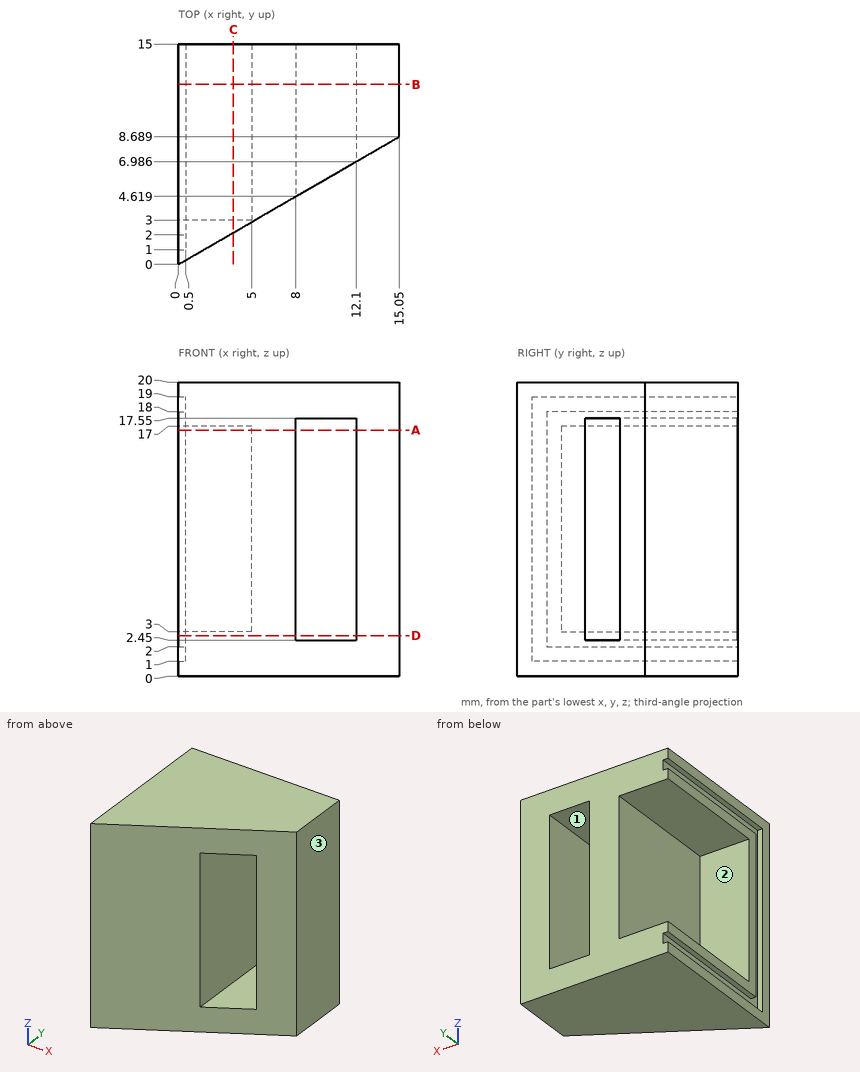
Answer from the drawing. Dimensions are ordinates in mm from the lowest x, y and z of the part. A direction names the side the tool comes from. Coordinates: 2 decimals unless noted, no trailing zeros. Loops run counter-clockwise (first coordinate to the right, second up) from the corner with the lowest first, then second, coordinate; pieces in that order, holes last. Notation, with made-up numbers: (-3, -32.5) - (35, -32.5) arc R8 ccw to (35, -22.5) - close; hole circle Ø8 at (-29, -4.75). An arc over 180 degrees is marked (long way). Answer in a Markdown table with one row per item.
1. Which of the six approach directions +Z, -Z, +X, -X, +Y, -Y give full straight-line access (tool end or side, diameter ignored) to the marked faces 1, 2 and 3?
Conclusion:
| item | result |
|---|---|
| face 1 | +Y, -Y |
| face 2 | -X, +Y |
| face 3 | +Z, -Z, +X, +Y, -Y |
2. Find section C-C, the plane x = 3.75. Write down the section's boundary in (y, z) (3 decimals), then the cut area to 3 significant figures.
Conclusion:
| item | result |
|---|---|
| outline | (2.165, 0) - (15, 0) - (15, 3) - (3, 3) - (3, 17) - (15, 17) - (15, 20) - (2.165, 20) - close |
| area | 88.7 mm² |
3. Given pin 1 (1 mm diameter, centred on y = 3, z = 3, fed in from -X); pin 2 (6.5 mm diameter, centred on y = 9.5, z = 13.5, fed in from -X); pin 3 (2 mm diameter, centred on x = 3, z = 12.5, fed in from +Y); pin 4 (1 mm diameter, centred on y = 2.5, z = 12.5, fed in from +X) (1 decimal), each flat-ended and moving along its own axis, determine where each tip first touches the part or whether it passes through.
Conclusion:
| item | result |
|---|---|
| pin 1 | stops at x = 0 |
| pin 2 | stops at x = 5 |
| pin 3 | stops at y = 3 |
| pin 4 | stops at x = 5.2 |
4. Straight lines are drawn through the part: line 1 (Z direction, x = 3.25, y = 4); line 2 (X direction, y = 11.5, z = 7); line 3 (Z direction, x = 11, y = 9). For each, find the intervals that lie inside material, in ascending order.
Conclusion:
| item | result |
|---|---|
| line 1 | z = 0 to 3, 17 to 20 |
| line 2 | x = 5 to 8, 12.1 to 15.05 |
| line 3 | z = 0 to 2.45, 17.55 to 20 |
5. Find section B-B, the plane y = 12.25. Write down the section's boundary in (x, z).
Conclusion:
| item | result |
|---|---|
| outline | (0, 0) - (15.05, 0) - (15.05, 20) - (0, 20) - (0, 19) - (0.5, 19) - (0.5, 18) - (0, 18) - (0, 17) - (5, 17) - (5, 3) - (0, 3) - (0, 2) - (0.5, 2) - (0.5, 1) - (0, 1) - close; hole (8, 2.45) - (12.1, 2.45) - (12.1, 17.55) - (8, 17.55) - close |
6. Find section A-A, the plane z = 16.75. Write down the section's boundary in (x, y).
Conclusion:
| item | result |
|---|---|
| outline | (0, 0) - (8, 4.62) - (8, 15) - (5, 15) - (5, 3) - (0, 3) - (0, 2) - (0.5, 2) - (0.5, 1) - (0, 1) - close; (12.1, 6.99) - (15.05, 8.69) - (15.05, 15) - (12.1, 15) - close |
7. Find section D-D, the plane z = 2.75. Write down the section's boundary in (x, y), then the cut area to 3 significant figures.
Conclusion:
| item | result |
|---|---|
| outline | (0, 0) - (8, 4.62) - (8, 15) - (0, 15) - (0, 2) - (0.5, 2) - (0.5, 1) - (0, 1) - close; (12.1, 6.99) - (15.05, 8.69) - (15.05, 15) - (12.1, 15) - close |
| area | 122 mm² |
